Read the model definition and answer for the solid it produces. Units are mm, in the model's axes. Face numbers are marked on the shaded views. Give positions to 0.01 mm unless a question says otherwise; leave off trailing zeros. Order: outer loops, then holes, each group sorted by start corner. A loop starts at its lowest first (then second) coordinate and runs counter-clockwise, first axis right, second up. Notation, with made-up numbers: (47.5, -34.5) -> (75.5, -34.5) arc R12 ccw to (75.5, -11.5) -> close; hole circle Ø4 at (79, 37). An arc over 180 degrees is marked (long way). Use one line per item in the form item = value.
```python
from build123d import *

# Parameters (mm, degrees)
SKETCH_1_W               = 23
SKETCH_1_H               = 15
EXTRUDE_1_DEPTH          = 0.5
OTHER_START              = -7.5
OTHER_1_DEPTH            = 15
OTHER_1_2_DEPTH          = 15
SM_START                 = -7.5
SM_EDGE_FLANGE_1_DEPTH   = 15
SM_EDGE_FLANGE_1_2_DEPTH = 15
FILLET_1_R               = 2
SKETCH_16_R              = 1.5
CUT_EXTRUDE_1_DEPTH      = 10


# Read off the part's stored shape, not the designer's step: Нарисованный сгиб1, Ребро-кромка1
with BuildPart() as part:
    # Sketch 1 → Бобышка-Вытянуть1 (new body)
    with BuildSketch(Plane(origin=(0, 0, 0), x_dir=(1, 0, 0), z_dir=(0, 1, 0))):
        with Locations((-9.5, 0)):
            Rectangle(SKETCH_1_W, SKETCH_1_H)
    extrude(amount=EXTRUDE_1_DEPTH)

    # Other 1 outline → Other 1 (cut)
    with BuildSketch(Plane.XY.offset(OTHER_START)):
        with BuildLine():
            ThreePointArc((0.042587685, 0), (-0.994234383, 0.126871677), (-1.969873495, 0.5))
            Line((-1.969873495, 0.5), (-21, 0.5))
            Line((-21, 0.5), (-21, 0))
            Line((-21, 0), (0.042587685, 0))
        make_face()
    extrude(amount=OTHER_1_DEPTH, mode=Mode.SUBTRACT)

    # Other 1 2 outline → Other 1 2 (add)
    with BuildSketch(Plane.XY.offset(OTHER_START)):
        with BuildLine():
            ThreePointArc((0.042587685, 0.5), (-2.644418083, 6.987005769), (3.842587685, 4.3))
            Line((3.842587685, 4.3), (3.842587685, 2.342587685))
            Line((3.842587685, 2.342587685), (4.342587685, 2.342587685))
            Line((4.342587685, 2.342587685), (4.342587685, 4.3))
            ThreePointArc((4.342587685, 4.3), (-2.175115736, 7.983991251), (-1.969873495, 0.5))
            Line((-1.969873495, 0.5), (0.042587685, 0.5))
        make_face()
    extrude(amount=OTHER_1_2_DEPTH)

    # Ребро-кромка1 outline → Ребро-кромка1 (cut)
    with BuildSketch(Plane.XY.offset(SM_START)):
        with BuildLine():
            ThreePointArc((1.085786438, 0.5), (1.46846987, 0.423879533), (1.792893219, 0.207106781))
            Line((1.792893219, 0.207106781), (2, 0))
            Line((2, 0), (2, 0.5))
            Line((2, 0.5), (1.085786438, 0.5))
        make_face()
        with BuildLine():
            Line((3.842587685, 2.342587685), (4.342587685, 2.342587685))
            Line((4.342587685, 2.342587685), (4.135480904, 2.549694466))
            ThreePointArc((4.135480904, 2.549694466), (3.918708153, 2.874117815), (3.842587685, 3.256801248))
            Line((3.842587685, 3.256801248), (3.842587685, 2.342587685))
        make_face()
    extrude(amount=SM_EDGE_FLANGE_1_DEPTH, mode=Mode.SUBTRACT)

    # Sm Edge Flange 1 2 outline → Sm Edge Flange 1 2 (add)
    with BuildSketch(Plane.XY.offset(SM_START)):
        with BuildLine():
            Line((6.449747468, -4.449747468), (2, 0))
            Line((2, 0), (1.085786438, 0))
            ThreePointArc((1.085786438, 0), (1.277128154, -0.038060234), (1.439339828, -0.146446609))
            Line((1.439339828, -0.146446609), (6.096194078, -4.803300859))
            Line((6.096194078, -4.803300859), (6.449747468, -4.449747468))
        make_face()
        with BuildLine():
            Line((8.792335154, -2.107159783), (9.145888544, -1.753606392))
            Line((9.145888544, -1.753606392), (4.489034295, 2.903247857))
            ThreePointArc((4.489034295, 2.903247857), (4.380647919, 3.065459531), (4.342587685, 3.256801248))
            Line((4.342587685, 3.256801248), (4.342587685, 2.342587685))
            Line((4.342587685, 2.342587685), (8.792335154, -2.107159783))
        make_face()
    extrude(amount=SM_EDGE_FLANGE_1_2_DEPTH)

    # Скругление1
    fillet_1_edges = [part.edges().sort_by_distance(p)[0] for p in [
        (8.969111849, -1.930383088, 7.5),
        (8.969111849, -1.930383088, -7.5),
        (6.272970773, -4.626524164, -7.5),
        (6.272970773, -4.626524164, 7.5),
    ]]
    fillet(fillet_1_edges, radius=FILLET_1_R)

    # Эскиз16 → Вырез-Вытянуть1 (cut)
    with BuildSketch(Plane(origin=(3.696141076, 3.696141076, 0), x_dir=(0, 0, -1), z_dir=(0.7071067811865587, 0.7071067811865365, 0))):
        with Locations(Location((2.46, -4.937106781, 0), (0, 0, 90))):
            Circle(SKETCH_16_R)
        with Locations(Location((-3.5, -3.707106781, 0), (0, 0, 90))):
            Circle(SKETCH_16_R)
    extrude(amount=-CUT_EXTRUDE_1_DEPTH, mode=Mode.SUBTRACT)


solid = part.part
```
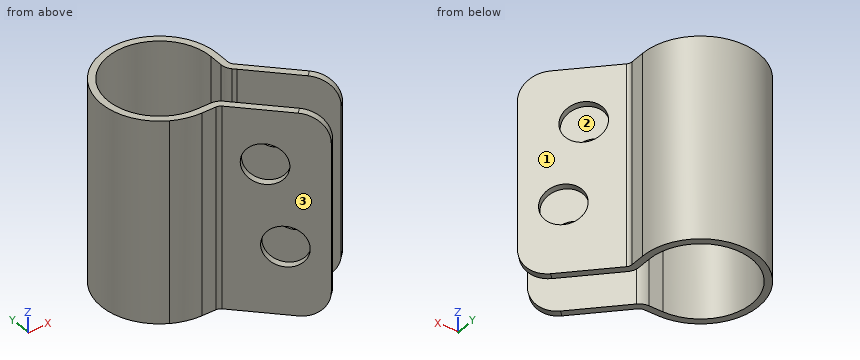
Item 1: The part is cut by section B-B on z = -1.25. Give the vertices of the cut face in (x, y).
Checks:
outline = (0.04, 0) -> (1.09, 0) arc R0.5 cw to (1.44, -0.15) -> (3.51, -2.22) -> (3.86, -1.86) -> (1.79, 0.21) arc R1 ccw to (1.09, 0.5) -> (0.04, 0.5) arc R3.8 cw (long way) to (3.84, 4.3) -> (3.84, 3.26) arc R1 ccw to (4.14, 2.55) -> (6.21, 0.48) -> (6.56, 0.83) -> (4.49, 2.9) arc R0.5 cw to (4.34, 3.26) -> (4.34, 4.3) arc R4.3 ccw (long way) to start; (4.76, -3.47) -> (6.1, -4.8) -> (6.45, -4.45) -> (5.12, -3.12) -> close; (7.46, -0.78) -> (8.79, -2.11) -> (9.15, -1.75) -> (7.81, -0.42) -> close
Item 2: The part is cut by section C-C on z = 1.5. Give the vertices of the cut face in (x, y).
Checks:
outline = (0.04, 0) -> (1.09, 0) arc R0.5 cw to (1.44, -0.15) -> (6.1, -4.8) -> (6.45, -4.45) -> (1.79, 0.21) arc R1 ccw to (1.09, 0.5) -> (0.04, 0.5) arc R3.8 cw (long way) to (3.84, 4.3) -> (3.84, 3.26) arc R1 ccw to (4.14, 2.55) -> (8.79, -2.11) -> (9.15, -1.75) -> (4.49, 2.9) arc R0.5 cw to (4.34, 3.26) -> (4.34, 4.3) arc R4.3 ccw (long way) to start
Item 3: Given pin 1 Ø4.5 at (x, y) = (0.04, 4.3) entering from +Z; pin 2 Ø1.5 at (x, z) = (2, -0.5) entering from +Y; pin 3 Ø0.8 at (y, z) = (3.5, -2) entering from +X; pin 4 Ø0.5 at (x, z) = (0.5, 0) entering from -Y, each flat-ended and moving along its own axis, determine where each tip first touches the part or whether it passes through.
Checks:
pin_1 = through
pin_2 = 8.43
pin_3 = 4.37
pin_4 = 0
Item 4: The part is cut by section A-A on x = -2.25. Give the vertices of the cut face in (y, z), and give its area (3 significant figures).
Checks:
outline = (0.66, -7.5) -> (1.27, -7.5) -> (1.27, 7.5) -> (0.66, 7.5) -> close; (7.33, -7.5) -> (7.94, -7.5) -> (7.94, 7.5) -> (7.33, 7.5) -> close
area = 18.2 mm²
Item 5: The part is cut by section D-D on x = -0.5. Give the vertices of the cut face in (y, z), and give its area (3 significant figures).
Checks:
outline = (0.03, -7.5) -> (0.54, -7.5) -> (0.54, 7.5) -> (0.03, 7.5) -> close; (8.06, -7.5) -> (8.57, -7.5) -> (8.57, 7.5) -> (8.06, 7.5) -> close
area = 15.1 mm²
Item 6: Straight lines are drawn through the part: L1, parallel to Y at x = 0.5, z = -2.75; L2, parallel to Y at x = 1.25, z = -5.5; L3, parallel to X at y = 7.25, z = 3.25. For each, find the intervals that lie inside material, in ascending order. Write a range as from..to.
Checks:
L1 = 0..0.5, 8.07..8.58
L2 = -0.03..0.49, 7.9..8.43
L3 = -3.09..-2.35, 2.44..3.17
Item 7: Determine the mould class of the marked faces 1, 2 and 3 for opening direction Y: +Y half, -Y half, draft (parallel to the pull), parting line (faces both ways), or undercut.
Checks:
face_1 = +Y half
face_2 = undercut
face_3 = -Y half
